Could you check a few things on this model? Use its own coordinates, in mm. A direction names the side the tool comes from. Coordinates: 2 decimals unless noted, no trailing zeros. Loops run counter-clockwise (first coordinate to the right, second up) from the corner with the lowest first, then second, coordinate; pieces in that order, holes last.
1) If I drill on line 1 along Y through (x, z) = (0, 22.35); line 2 along Z through (x, y) = (1.15, 0.9); line 3 along Z through (x, y) = (0.85, 1.5), over which ranges is the centre line in solid material (lowest first)?
2) Will these pins go through, and if not, where does the flat tip stop? P1, Ø1, axis at y = -1, z = 7, coming from the +X side; P2, Ø2, axis at y = -0.5, z = 18, coming from the -X side.
3) Imagine slicing it at D-D on z = 18. Please give me the cut outline in (x, y), plus the area to 3 significant figures.
4) Thinking about a two-plate mould opening in X: for faces 1 (the face through (-1.43, 0.45, -2.96)), 2 (the face through (1.51, -0.85, 12.32)), 3 (the face through (0, 0, 20)), which applies, released by +X, released by -X, zero draft, split by the parting line, or undercut?
5) For faces 4 (the face through (1.5, 0.07, 22.46)), 5 (the face through (0, 1.732, 12)), which set-ups out of +Z, -Z, +X, -X, +Y, -Y let a thin tool reach every point of the face, with its end or its side?
6) Imagine slicing it at B-B on y = -1.05. Please give me the cut outline in (x, z).
7) Imagine slicing it at C-C on x = 0.65. Please give me the cut outline in (y, z), plus the area to 3 significant figures.
8) Imagine slicing it at A-A on z = 22. Please give me the cut outline in (x, y), plus the area to 3 significant figures.
```python
from build123d import *

# Parameters (mm, degrees)
EXTRUDE_1_DEPTH           = 25
SKETCH_2_W                = 1.5
SKETCH_2_H                = 6
HOLE_WIZARD_3_0_3_1_D     = 3
HOLE_WIZARD_3_0_3_1_DEPTH = 5


with BuildPart() as part:
    # 草图1 → 凸台-拉伸1 (new body)
    with BuildSketch(Plane(origin=(0, 0, 0), x_dir=(-1, 0, 0), z_dir=(0, 0, -1))):
        Polygon((1, -1.732050808), (2, 0), (1, 1.732050808), (-1, 1.732050808), (-2, 0), (-1, -1.732050808), align=None)
    extrude(amount=-EXTRUDE_1_DEPTH)

    # 草图2 → 旋转1 (revolve)
    with BuildSketch(Plane.XZ, mode=Mode.PRIVATE) as revolve_1_sk:
        with Locations((0.75, -3)):
            Rectangle(SKETCH_2_W, SKETCH_2_H)
    revolve(revolve_1_sk.sketch.rotate(Axis((0, 0, 0), (0, 0, -1)), 180), axis=Axis((0, 0, 0), (0, 0, -1)))

    # Ø3.0 (3) 直径孔1
    with Locations(Plane.XY.offset(25)):
        with Locations((0, 0)):
            Hole(HOLE_WIZARD_3_0_3_1_D / 2, depth=HOLE_WIZARD_3_0_3_1_DEPTH)


solid = part.part
```
Filled in:
1. line 1: y = -1.73 to -1.5, 1.5 to 1.73
1. line 2: z = -6 to 20
1. line 3: z = 0 to 25
2. P1: stops at x = 1.71
2. P2: stops at x = -2
3. outline: (-2, 0) - (-1, -1.73) - (1, -1.73) - (2, 0) - (1, 1.73) - (-1, 1.73) - close
3. area: 10.4 mm2
4. face 1: split by the parting line
4. face 2: released by +X
4. face 3: undercut
5. face 4: +Z
5. face 5: +Z, -Z, +X, -X, +Y
6. outline: (-1.39, 0) - (-1.07, 0) - (-1.07, -6) - (1.07, -6) - (1.07, 0) - (1.39, 0) - (1.39, 25) - (1.07, 25) - (1.07, 20) - (-1.07, 20) - (-1.07, 25) - (-1.39, 25) - close
7. outline: (-1.73, 0) - (-1.35, 0) - (-1.35, -6) - (1.35, -6) - (1.35, 0) - (1.73, 0) - (1.73, 25) - (1.35, 25) - (1.35, 20) - (-1.35, 20) - (-1.35, 25) - (-1.73, 25) - close
7. area: 89.3 mm2
8. outline: (-2, 0) - (-1, -1.73) - (1, -1.73) - (2, 0) - (1, 1.73) - (-1, 1.73) - close; hole circle Ø3 at (0, 0)
8. area: 3.32 mm2
